from build123d import *

# Parameters (mm, degrees)
PAD003_DEPTH    = 4.7
CHAMFER001_SIZE = 0.1
PAD010_DEPTH    = 3.47
SKETCH019_W     = 0.2
SKETCH019_H     = 1.5
SKETCH019_H_2   = 1.3
PAD012_DEPTH    = 2.17
CHAMFER002_SIZE = 0.3


with BuildPart() as part:
    # Sketch002 → Pad003 (new body)
    with BuildSketch(Plane.XZ):
        with BuildLine():
            ThreePointArc((-2.89, 1.48), (-4.37, 0), (-2.89, -1.48))
            Line((-2.89, -1.48), (2.89, -1.48))
            ThreePointArc((2.89, -1.48), (4.37, 0), (2.89, 1.48))
            Line((-2.89, 1.48), (2.89, 1.48))
        make_face()
        with BuildLine():
            ThreePointArc((-2.89, 1.28), (-4.17, 0), (-2.89, -1.28))
            Line((-2.89, -1.28), (2.89, -1.28))
            ThreePointArc((2.89, -1.28), (4.17, 0), (2.89, 1.28))
            Line((-2.89, 1.28), (2.89, 1.28))
        make_face(mode=Mode.SUBTRACT)
    extrude(amount=-PAD003_DEPTH)

    # Chamfer001
    chamfer001_edges = [part.edges().sort_by_distance(p)[0] for p in [
        (0, 4.7, 1.28),
    ]]
    chamfer(chamfer001_edges, length=CHAMFER001_SIZE)

    # Sketch014 → Pad010 (join)
    with BuildSketch(Plane.XZ):
        with BuildLine():
            ThreePointArc((-2.89, 1.48), (-4.37, 0), (-2.89, -1.48))
            Line((-2.89, -1.48), (2.89, -1.48))
            ThreePointArc((2.89, -1.48), (4.37, 0), (2.89, 1.48))
            Line((-2.89, 1.48), (2.89, 1.48))
        make_face()
    extrude(amount=PAD010_DEPTH)

    # Sketch019 → Pad012 (join)
    with BuildSketch(Plane.XY):
        with Locations((-4.27, 2.4)):
            Rectangle(SKETCH019_W, SKETCH019_H)
        with Locations((-4.27, -2.65)):
            Rectangle(SKETCH019_W, SKETCH019_H_2)
    pad012 = extrude(amount=-PAD012_DEPTH)

    # Mirrored002: Pad012 across Sketch019 V_Axis
    add(pad012.mirror(Plane(origin=(0, 0, 0), x_dir=(0, 0, 1), z_dir=(1, 0, 0))))

    # Chamfer002
    chamfer002_edges = [part.edges().sort_by_distance(p)[0] for p in [
        (4.27, -3.3, -2.17),
        (4.27, -2, -2.17),
        (4.27, 1.65, -2.17),
        (4.27, 3.15, -2.17),
        (-4.27, -3.3, -2.17),
        (-4.27, -2, -2.17),
        (-4.27, 1.65, -2.17),
        (-4.27, 3.15, -2.17),
    ]]
    chamfer(chamfer002_edges, length=CHAMFER002_SIZE)


solid = part.part
Build history of the part. All positions in model axes, mm. A direction names the side the tool comes from. Give positions to 0.01 mm unless a question says otherwise; leave off trailing zeros. Order: outer loops, then holes, each group sorted by start corner. A loop starts at its lowest first (then second) coordinate and runs counter-clockwise, first axis right, second up. Notation, with made-up numbers: M 86.25,14.5 L 124.25,14.5 A23 cw 124.25,52.5 Z; hole C 74,-27 d10. An arc over 180 degrees is marked long. Use one line per item in the form item = value.
1) Tool access for faces 4 (the face through (0, 1, -1.48)), 5 (the face through (0, -3.47, 0)), 6 (the face through (4.17, 2.27, -0.03)): list every direction of +Z, -Z, +X, -X, +Y, -Y with a clear straight run to the whole face (end or side of a thin tool).
Calculated:
face_4 = -Z, +Y, -Y
face_5 = +Z, -Z, +X, -X, -Y
face_6 = +Y
2) Drop flat-ended pins along their axis: pin 1 (2 mm diameter, centred on y = 2, z = 0.5, fed in from -X); pin 2 (1.7 mm diameter, centred on x = 1, y = 2.5, fed in from -Z); pin 3 (1.3 mm diameter, centred on x = -1, z = 0, fed in from +Y). Give the stop position or say it passes through.
Calculated:
pin_1 = -4.37
pin_2 = -1.48
pin_3 = 0
3) Probe probe 1 along Z at (x, y) = (1.75, -0.5); probe 2 along X at (y, z) = (4, -0.5); probe 3 along X at (y, z) = (2.5, -0.3). List the from-to ranges inside material, lowest first.
Calculated:
probe_1 = -1.48 to 1.48
probe_2 = -4.28 to -4.07, 4.07 to 4.28
probe_3 = -4.37 to -4.13, 4.13 to 4.37
4) Saw through at C-C (y = 2.5). Give the cut face in (x, z).
Calculated:
outline = M -4.37,-2.17 L -4.17,-2.17 L -4.17,-0.74 A1.48 ccw -2.89,-1.48 L 2.89,-1.48 A1.48 ccw 4.17,-0.74 L 4.17,-2.17 L 4.37,-2.17 L 4.37,0 A1.48 ccw 2.89,1.48 L -2.89,1.48 A1.48 ccw -4.37,0 Z; hole M -2.89,-1.28 L 2.89,-1.28 A1.28 ccw 2.89,1.28 L -2.89,1.28 A1.28 ccw Z
5) Saw through at B-B (x = 1.75). Give the cut face in (y, z), plus the area to 3 significant figures.
Calculated:
outline = M -3.47,-1.48 L 4.7,-1.48 L 4.7,-1.38 L 4.6,-1.28 L 0,-1.28 L 0,1.28 L 4.6,1.28 L 4.7,1.38 L 4.7,1.48 L -3.47,1.48 Z
area = 12.1 mm2
6) Saw through at A-A (y = 0.25). Give the cut face in (x, z).
Calculated:
outline = M -2.89,-1.48 L 2.89,-1.48 A1.48 ccw 2.89,1.48 L -2.89,1.48 A1.48 ccw Z; hole M -2.89,-1.28 L 2.89,-1.28 A1.28 ccw 2.89,1.28 L -2.89,1.28 A1.28 ccw Z
7) Two-plate mould, pull along Z, no slides. Class faces 1 (the face through (0, 2, 1.28)), 2 (the face through (4.37, -3, -1)), 3 (the face through (0, 1, 1.48)): released by +Z, released by -Z, zero draft, split by the parting line, or undercut.
Calculated:
face_1 = undercut
face_2 = zero draft
face_3 = released by +Z
8) Saw through at D-D (z = -0.95). State how many separate pieces and enclosed holes the cut face has, plus the area to 3 significant figures.
Calculated:
separate_pieces = 5
enclosed_holes = 0
area = 31.6 mm2
